```python
from build123d import *

# Parameters (mm, degrees)
SKETCH1_R           = 75
BOSS_EXTRUDE1_DEPTH = 4
SKETCH2_R           = 45
SKETCH2_R_2         = 40
BOSS_EXTRUDE2_DEPTH = 8
SKETCH4_R           = 3
CUT_EXTRUDE1_DEPTH  = 13


with BuildPart() as part:
    # Sketch1 → Boss-Extrude1 (new body)
    with BuildSketch(Plane.XY):
        Circle(SKETCH1_R)
    extrude(amount=BOSS_EXTRUDE1_DEPTH)

    # Sketch2 → Boss-Extrude2 (add)
    with BuildSketch(Plane.XY.offset(4)):
        Circle(SKETCH2_R)
        Circle(SKETCH2_R_2, mode=Mode.SUBTRACT)
    extrude(amount=BOSS_EXTRUDE2_DEPTH)

    # Sketch4 → Cut-Extrude1 (cut, through all)
    with BuildSketch(Plane(origin=(0, 0, 0), x_dir=(-1, 0, 0), z_dir=(0, 0, -1))):
        with Locations((0, 60)):
            Circle(SKETCH4_R)
        with Locations((51.961524227, -30)):
            Circle(SKETCH4_R)
        with Locations((-51.961524227, -30)):
            Circle(SKETCH4_R)
    extrude(amount=-CUT_EXTRUDE1_DEPTH, mode=Mode.SUBTRACT)


solid = part.part
```
Source: CAD feature listing. Evaluate the final solid. Frame: model axes, mm. A direction names the side the tool comes from. Coordinates: 2 decimals unless noted, no trailing zeros. Write each loop counter-clockwise with the first axis right and the second up, starting at its lowest first coordinate (ties: lowest second). Pieces come first, ordered by that corner, then holes. Notation, with made-up numbers: M 14.25,-3.75 L 26.25,-3.75 A5 cw 26.25,1.25 Z; hole C -28.5,-7 d4. An arc over 180 degrees is marked long. Answer as a JSON object with one key per item and string values.
1. Draft query along Y for faces 1 (the cylindrical face through (0, 63, 2)), 2 (the cylindrical face through (-9.764, 74.362, 1.972)), 3 (the flat face through (32, -32, 4)). Return one class per face: released by +Y, released by -Y, zero draft, split by the parting line, or undercut.
Evaluation:
{"face 1": "undercut", "face 2": "split by the parting line", "face 3": "zero draft"}
2. Cut plane A-A on y = 60. Output: boundary loops of the cut face in (x, z).
Evaluation:
{"outline": "M -45,0 L -3,0 L -3,4 L -45,4 Z; M 3,0 L 45,0 L 45,4 L 3,4 Z"}
3. Cut plane D-D on z = 9.25. Output: boundary loops of the cut face in (x, y).
Evaluation:
{"outline": "C 0,0 d90; hole C 0,0 d80"}
4. Cut plane C-C on y = -30. Output: boundary loops of the cut face in (x, z), plus the area to 3 significant figures.
Evaluation:
{"outline": "M -68.74,0 L -54.96,0 L -54.96,4 L -68.74,4 Z; M -48.96,0 L 48.96,0 L 48.96,4 L 33.54,4 L 33.54,12 L 26.46,12 L 26.46,4 L -26.46,4 L -26.46,12 L -33.54,12 L -33.54,4 L -48.96,4 Z; M 54.96,0 L 68.74,0 L 68.74,4 L 54.96,4 Z", "area": "615 mm^2"}
5. Contact query for flat-ended pins moving along their axis: P1, Ø4, axis at y = -15, z = 9, coming from the +X side; P2, Ø24, axis at x = -12, y = -20, coming from the +Z side; P3, Ø2, axis at y = 7.5, z = 4.5, coming from the +X side. Output: stop coordinate, or through.
Evaluation:
{"P1": "x = 43.08", "P2": "z = 4", "P3": "x = 74.71"}
6. Cut plane B-B on x = 0. Output: boundary loops of the cut face in (y, z), plus the area to 3 significant figures.
Evaluation:
{"outline": "M -75,0 L 57,0 L 57,4 L 45,4 L 45,12 L 40,12 L 40,4 L -40,4 L -40,12 L -45,12 L -45,4 L -75,4 Z; M 63,0 L 75,0 L 75,4 L 63,4 Z", "area": "656 mm^2"}
7. Ray query, L1, parallel to Y at x = 0, z = 6.25; L2, parallel to Y at x = 0, z = 2.65; L3, parallel to X at y = -1, z = 11.25. Return the intervals inside material, ascending.
Evaluation:
{"L1": "-45 to -40, 40 to 45", "L2": "-75 to 57, 63 to 75", "L3": "-44.99 to -39.99, 39.99 to 44.99"}
8. Access query for faces 4 (the cylindrical face through (-54.823, -29.099, 1.972)), 5 (the cylindrical face through (20.765, -39.923, 7.944)). Directions: +Z, -Z, +X, -X, +Y, -Y. A direction counts if a zero-diameter tool reaches every point of the face in a straight line with its end or side. Return the directions, or none.
Evaluation:
{"face 4": "+Z, -Z", "face 5": "+Z"}
